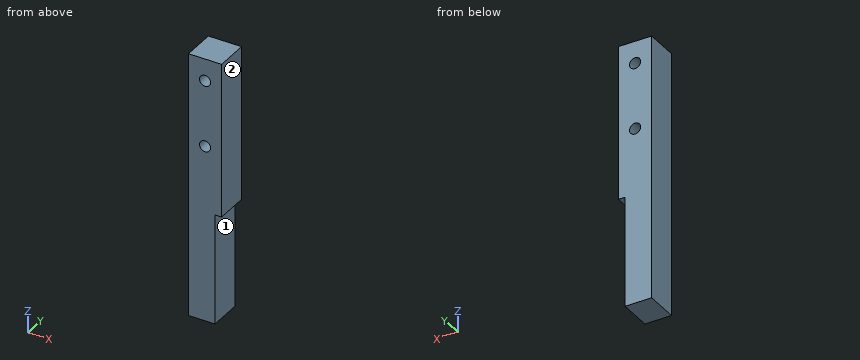
from build123d import *

# Parameters (mm, degrees)
SKETCH1_W           = 19.05
SKETCH1_H           = 19.05
BOSS_EXTRUDE1_DEPTH = 152.4
SKETCH3_R           = 3.175
SKETCH3_W           = 3.81
SKETCH3_H           = 63.5
CUT_EXTRUDE1_DEPTH  = 25.4


with BuildPart() as part:
    # Sketch1 → Boss-Extrude1 (new body)
    with BuildSketch(Plane.XY):
        Rectangle(SKETCH1_W, SKETCH1_H)
    extrude(amount=BOSS_EXTRUDE1_DEPTH)

    # Sketch3 → Cut-Extrude1 (cut)
    with BuildSketch(Plane.XZ.offset(9.525)):
        with Locations(Location((0, 139.7, 0), (0, 0, 270))):
            Circle(SKETCH3_R)
        with Locations(Location((0, 101.6, 0), (0, 0, 270))):
            Circle(SKETCH3_R)
        with Locations((7.62, 31.75)):
            Rectangle(SKETCH3_W, SKETCH3_H)
    extrude(amount=-CUT_EXTRUDE1_DEPTH, mode=Mode.SUBTRACT)


solid = part.part
Read the model definition and answer for the solid it produces. Units are mm, in the model's axes. Face numbers are marked on the shaded views. A direction names the side the tool comes from. Coordinates: 2 decimals unless noted, no trailing zeros. Loops run counter-clockwise (first coordinate to the right, second up) from the corner with the lowest first, then second, coordinate; pieces in that order, holes last.
Q1. Each of these flat-tipped pins is pushed along its axis until it touches: pin 1 Ø5 at (x, z) = (0, 139.7) entering from -Y; pin 2 Ø8 at (y, z) = (5, 16) entering from +X (3 decimals); pin 3 Ø7.5 at (x, z) = (0, 101.6) entering from -Y (3 decimals); pin 4 Ø1.1 at (x, y) = (7, -2) entering from -Z. Where does it stop, or does it pass through?
Q2. The part is cut by section A-A on x = 0. Write down the section's boundary in (y, z) (3 decimals), and give its area (3 significant figures).
Q3. Which of the six approach directions +Z, -Z, +X, -X, +Y, -Y give full straight-line access (tool end or side, diameter ignored) to the marked faces 1 and 2?
Q4. Consider probe 1 along X at (y, z) = (-1, 139.7) (3 decimals); probe 2 along Z at (x, y) = (-0.5, 6.5); probe 3 along Z at (x, y) = (6, 2.25). Determine where each line is inside the solid, lowest interval first.
Q5. The part is cut by section D-D on z = 60. Write down the section's boundary in (x, y) (3 decimals).
Q6. The part is cut by section B-B on y = -5.25. Write down the section's boundary in (x, z) (3 decimals).
Q7. The part is cut by section C-C on z = 101.6. Write down the section's boundary in (x, y) (3 decimals), and give its area (3 significant figures).
Results below:
1. pin 1: passes through
1. pin 2: stops at x = 5.715
1. pin 3: stops at y = -9.525
1. pin 4: stops at z = 63.5
2. outline: (-9.525, 0) - (9.525, 0) - (9.525, 98.425) - (-9.525, 98.425) - close; (-9.525, 104.775) - (9.525, 104.775) - (9.525, 136.525) - (-9.525, 136.525) - close; (-9.525, 142.875) - (9.525, 142.875) - (9.525, 152.4) - (-9.525, 152.4) - close
2. area: 2,660 mm2
3. face 1: -Z, +X, +Y, -Y
3. face 2: +Z, -Z, +X, +Y, -Y
4. probe 1: x = -9.525 to -3.175, 3.175 to 9.525
4. probe 2: z = 0 to 98.46, 104.74 to 136.56, 142.84 to 152.4
4. probe 3: z = 63.5 to 152.4
5. outline: (-9.525, -9.525) - (5.715, -9.525) - (5.715, 9.525) - (-9.525, 9.525) - close
6. outline: (-9.525, 0) - (5.715, 0) - (5.715, 63.5) - (9.525, 63.5) - (9.525, 152.4) - (-9.525, 152.4) - close; hole circle Ø6.35 at (0, 101.6); hole circle Ø6.35 at (0, 139.7)
7. outline: (-9.525, -9.525) - (-3.175, -9.525) - (-3.175, 9.525) - (-9.525, 9.525) - close; (3.175, -9.525) - (9.525, -9.525) - (9.525, 9.525) - (3.175, 9.525) - close
7. area: 242 mm2
